Source: CAD feature listing. Evaluate the final solid. Frame: model axes, mm. Give positions to 0.01 mm unless a question says otherwise; leave off trailing zeros. Order: outer loops, then holes, each group sorted by start corner. A loop starts at its lowest first (then second) coordinate and runs counter-clockwise, first axis right, second up.
1) Draft query along Z for faces 1 (the face through (-1, 0, 21)), 2 (the face through (14.539, -95.243, 4.579)), 3 (the face through (48, -51, 49)). Return one class per face: released by +Z, released by -Z, zero draft, split by the parting line, or undercut.
2) Section C-C, the plane x = 0. Return loops of the section in (y, z), plus the area to 3 significant figures.
3) Section D-D, the plane x = 36. Return loops of the section in (y, z), plus the area to 3 significant figures.
4) Material intervals for line 1 (Z direction, x = 0, y = -71); line 2 (Y direction, x = -35.5, z = 0), sorted ascending.
5) Section A-A, the plane z = 0. Return loops of the section in (x, y).
6) Section B-B, the plane y = -76.5. Return loops of the section in (x, z).
```python
from build123d import *

# Parameters (mm, degrees)
F0_W     = 100
F0_H     = 100
F0_R     = 15
F1_DEPTH = 100
F2_R     = 15
F3_DEPTH = 100
F4_R     = 15
F5_DEPTH = 100
F6_R     = 5
F7_SIZE  = 5


with BuildPart() as f1:
    # F0 (on Front) → F1 (new body)
    with BuildSketch(Plane.XZ):
        Rectangle(F0_W, F0_H)
        Circle(F0_R, mode=Mode.SUBTRACT)
    extrude(amount=F1_DEPTH)

    # F2 (on face) → F3 (cut)
    with BuildSketch(Plane.YZ.offset(50)):
        with Locations((-50.151795, 0)):
            Circle(F2_R)
    extrude(amount=-F3_DEPTH, mode=Mode.SUBTRACT)

    # F4 (on face) → F5 (cut)
    with BuildSketch(Plane.XY.offset(50)):
        with Locations((0, -50.267148)):
            Circle(F4_R)
    extrude(amount=-F5_DEPTH, mode=Mode.SUBTRACT)

    # F6
    f6_edges = [f1.edges().sort_by_distance(p)[0] for p in [
        (0, -100, 50),
        (50, -50, 50),
        (50, -100, 0),
        (0, -100, -50),
        (50, -50, -50),
        (50, 0, 0),
        (0, 0, 50),
        (-50, 0, 0),
        (0, 0, -50),
        (-50, -50, -50),
        (-50, -50, 50),
        (-50, -100, 0),
    ]]
    fillet(f6_edges, radius=F6_R)

    # F7
    f7_edges = [f1.edges().sort_by_distance(p)[0] for p in [
        (-15, -100, 0),
        (-15, -50.267148, 50),
        (50, -65.151795, 0),
        (-15, 0, 0),
        (-15, -50.267148, -50),
        (-50, -65.151795, 0),
    ]]
    chamfer(f7_edges, length=F7_SIZE)


solid = f1.part
```
From the geometry:
1. face 1: zero draft
1. face 2: undercut
1. face 3: released by +Z
2. outline: (-100, -45) arc R5 ccw to (-95, -50) - (-70.27, -50) - (-65.27, -45) - (-65.27, -15) - (-95, -15) - (-100, -20) - close; (-100, 20) - (-95, 15) - (-65.27, 15) - (-65.27, 45) - (-70.27, 50) - (-95, 50) arc R5 ccw to (-100, 45) - close; (-35.27, -45) - (-30.27, -50) - (-5, -50) arc R5 ccw to (0, -45) - (0, -20) - (-5, -15) - (-35.27, -15) - close; (-35.27, 15) - (-5, 15) - (0, 20) - (0, 45) arc R5 ccw to (-5, 50) - (-30.27, 50) - (-35.27, 45) - close
2. area: 4,780 mm2
3. outline: (-100, -45) arc R5 ccw to (-95, -50) - (-5, -50) arc R5 ccw to (0, -45) - (0, 45) arc R5 ccw to (-5, 50) - (-95, 50) arc R5 ccw to (-100, 45) - close; hole circle Ø30 at (-50.15, 0)
3. area: 9,270 mm2
4. line 1: z = -50 to -15, 15 to 50
4. line 2: y = -100 to -65.15, -35.15 to 0
5. outline: (-50, -95) arc R5 ccw to (-45, -100) - (-20, -100) - (-15, -95) - (-15, -65.15) - (-45, -65.15) - (-50, -70.15) - close; (-50, -30.15) - (-45, -35.15) - (-15, -35.15) - (-15, -5) - (-20, 0) - (-45, 0) arc R5 ccw to (-50, -5) - close; (15, -95) - (20, -100) - (45, -100) arc R5 ccw to (50, -95) - (50, -70.15) - (45, -65.15) - (15, -65.15) - close; (15, -35.15) - (45, -35.15) - (50, -30.15) - (50, -5) arc R5 ccw to (45, 0) - (20, 0) - (15, -5) - close
6. outline: (-50, -45) arc R5 ccw to (-45, -50) - (45, -50) arc R5 ccw to (50, -45) - (50, 45) arc R5 ccw to (45, 50) - (-45, 50) arc R5 ccw to (-50, 45) - close; hole circle Ø30 at (0, 0)
